from build123d import *

# Parameters (mm, degrees)
F1_R     = 18.923
F2_DEPTH = 50.8
F0_W     = 76.2
F0_H     = 152.4
F3_DEPTH = 6.35
F4_SIZE  = 5.08


with BuildPart() as f2:
    # F1 (on face) → F2 (new body)
    with BuildSketch(Plane.XZ):
        with Locations((0, 50.433476)):
            Circle(F1_R)
    extrude(amount=F2_DEPTH)

    # F0 (on Front) → F3 (join)
    with BuildSketch(Plane.XZ):
        Rectangle(F0_W, F0_H)
    extrude(amount=F3_DEPTH)

    # F4
    f4_edges = [f2.edges().sort_by_distance(p)[0] for p in [
        (-18.923, -50.8, 50.433476),
    ]]
    chamfer(f4_edges, length=F4_SIZE)


solid = f2.part
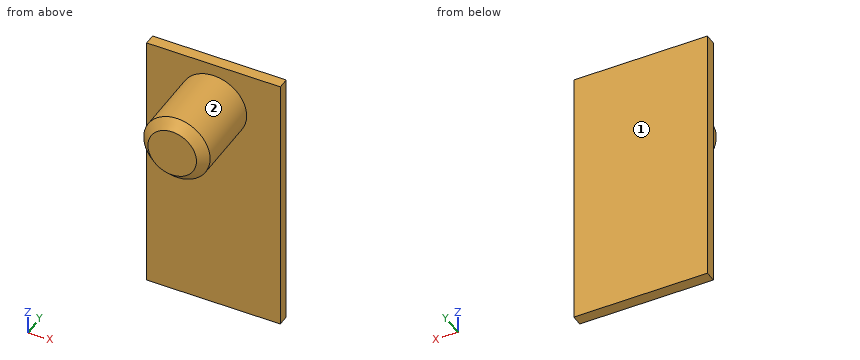
Check sheet for the modelled part. Datum: model origin and axes. Units: mm. Face numbers are marked on the shaded views. A direction names the side the tool comes from. Round coordinates to 2 decimals unless told otherwise and drop trailing zeros. Loops run counter-clockwise (first coordinate to the right, second up) from the corner with the lowest first, then second, coordinate; pieces in that order, holes last. Notation, with made-up numbers: (84, -39.5) -> (119, -39.5) arc R21 cw to (119, -9.5) -> close; hole circle Ø3 at (-15, -13.75). An arc over 180 degrees is marked (long way). Put each result on its own line as item: value. Start each with the question number.
1. Section check D-D (y = -28). Enter the section's corners in (x, z).
2. Section check B-B (z = -57). Enter the section's corners in (x, y), plus the area to 3 significant figures.
3. Scan lines: probe 1 along Y at (x, z) = (-14.5, 34); probe 2 along X at (y, z) = (-17, 54.5); probe 3 along X at (y, z) = (-7, 68). Record each from-to range of solid material in increasing order.
4. Gauge pin test, flat ends, axial feed: pin 1 (5 mm diameter, centred on x = 3, y = -13, fed in from -Z); pin 2 (4 mm diameter, centred on x = -27.5, z = 36, fed in from -Y); pin 3 (6 mm diameter, centred on x = -17.5, y = -38, fed in from -Z). Record the tip position at first contact, or that the pin passes through.
5. Section check A-A (x = 0). Enter the section's corners in (y, z).
6. Access from +Z, -Z, +X, -X, +Y, -Y to the whole of each face (thin tool, end or side, straight path). Record for the marked faces 1 and 2.
7. Section check C-C (x = 24). Enter the section's corners in (y, z), plus the area to 3 significant figures.
Findings:
1. outline: circle Ø37.85 at (0, 50.43)
2. outline: (-38.1, -6.35) -> (38.1, -6.35) -> (38.1, 0) -> (-38.1, 0) -> close
2. area: 484 mm^2
3. probe 1: y = -6.35 to 0
3. probe 2: x = -18.48 to 18.48
3. probe 3: x = -7.04 to 7.04
4. pin 1: stops at z = 31.52
4. pin 2: stops at y = -6.35
4. pin 3: stops at z = 38.27
5. outline: (-50.8, 36.59) -> (-45.72, 31.51) -> (-6.35, 31.51) -> (-6.35, -76.2) -> (0, -76.2) -> (0, 76.2) -> (-6.35, 76.2) -> (-6.35, 69.36) -> (-45.72, 69.36) -> (-50.8, 64.28) -> close
6. face 1: +Z, -Z, +X, -X, +Y
6. face 2: -Y
7. outline: (-6.35, -76.2) -> (0, -76.2) -> (0, 76.2) -> (-6.35, 76.2) -> close
7. area: 968 mm^2
